```python
from build123d import *

# Parameters (mm, degrees)
RESSALTO_EXTRUS_O2_DEPTH = 10
SKETCH1_R                = 1
SKETCH1_R_2              = 3
CUT_EXTRUDE1_DEPTH       = 85.442226256


with BuildPart() as part:
    # Esboço2 → Ressalto-extrusão2 (new body)
    with BuildSketch(Plane(origin=(0, 0, 0), x_dir=(0, 0, -1), z_dir=(1, 0, 0))):
        Polygon((67, -31.48985963), (75, -31.48985963), (75, -37.48985963), (-75, -37.48985963), (-75, -31.48985963), (-67, -31.48985963), (-67, -5.780687565), (-5.390847643, -0.390585164), (0, -0.390585164), (5.390847643, -0.390585164), (67, -5.780687565), align=None)
    extrude(amount=RESSALTO_EXTRUS_O2_DEPTH)

    # Sketch1 → Cut-Extrude1 (cut, through all)
    with BuildSketch(Plane.ZY):
        with Locations((-57, -29.48985963)):
            Circle(SKETCH1_R)
        with Locations(Location((57, -29.48985963, 0), (0, 0, 180))):
            Circle(SKETCH1_R)
        with Locations((0, -8.390585164)):
            Circle(SKETCH1_R)
        with Locations((0, -27.002843351)):
            Circle(SKETCH1_R_2)
        with Locations((-57, -13.178770397)):
            Circle(SKETCH1_R_2)
        with Locations((57, -13.178770397)):
            Circle(SKETCH1_R_2)
    extrude(amount=-CUT_EXTRUDE1_DEPTH, mode=Mode.SUBTRACT)


solid = part.part
```
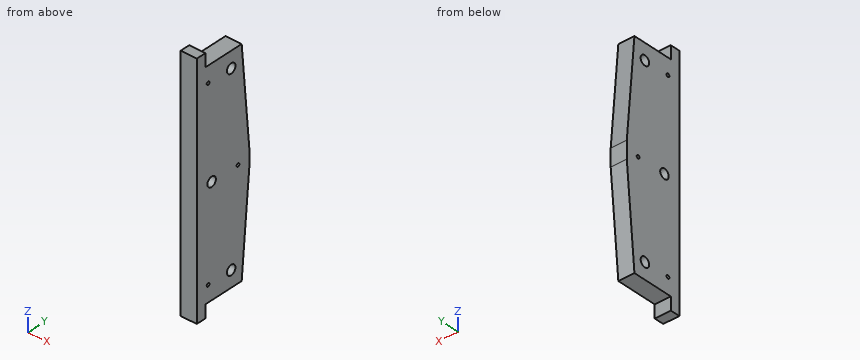
The model under review builds one solid part; all positions refer to its coordinate system, in mm. Round coordinates to 2 decimals unless told otherwise and drop trailing zeros. Loops run counter-clockwise (first coordinate to the right, second up) from the corner with the lowest first, then second, coordinate; pieces in that order, holes last. Notation, with made-up numbers: (-34.5, -26) - (-1.5, -26) arc R9 ccw to (-1.5, -12) - close; hole circle Ø10 at (70, -14). An arc over 180 degrees is marked (long way). Use a Markdown table: item, result. Add a question column.
Q1. For probe 1 along Y at (x, z) = (5.5, 0); probe 2 along Z at (x, y) = (5.5, -13.5); probe 3 along Y at (x, z) = (6.5, -57), list the stretches that pass through material, from the lowest coordinate up.
Q2. Insertion check: pin 1 Ø1.2 at (y, z) = (-8.39, 0) entering from +X; pin 2 Ø1.5 at (x, y) = (9, -24.5) entering from -Z; pin 3 Ø4 at (x, z) = (5.5, 71) entering from +Y. Each pin has a flat end and moves straight along its axis. Give the tip position at first contact, or say it passes through.
Q3. Add section C-C (z = 21.5). State the section outline as (x, y) points, plus the area to 3 significant figures.
Q4. Add section B-B (y = -17.5). State the section outline as (x, z) points.
Q5. Add section A-A (x = 1.25). State the section outline as (y, z) points, plus the area to 3 significant figures.
Worked answers:
| question | item | result |
|---|---|---|
| 1 | probe 1 | -37.49 to -30, -24 to -9.39, -7.39 to -0.39 |
| 1 | probe 2 | -67 to -59.98, -54.02 to 54.02, 59.98 to 67 |
| 1 | probe 3 | -37.49 to -30.49, -28.49 to -16.18, -10.18 to -4.91 |
| 2 | pin 1 | through |
| 2 | pin 2 | z = -67 |
| 2 | pin 3 | y = -31.49 |
| 3 | outline | (0, -37.49) - (10, -37.49) - (10, -1.8) - (0, -1.8) - close |
| 3 | area | 357 mm² |
| 4 | outline | (0, -67) - (10, -67) - (10, 67) - (0, 67) - close |
| 5 | outline | (-37.49, -75) - (-31.49, -75) - (-31.49, -67) - (-5.78, -67) - (-0.39, -5.39) - (-0.39, 5.39) - (-5.78, 67) - (-31.49, 67) - (-31.49, 75) - (-37.49, 75) - close; hole circle Ø2 at (-29.49, -57); hole circle Ø2 at (-29.49, 57); hole circle Ø6 at (-27, 0); hole circle Ø6 at (-13.18, -57); hole circle Ø6 at (-13.18, 57); hole circle Ø2 at (-8.39, 0) |
| 5 | area | 4,640 mm² |
